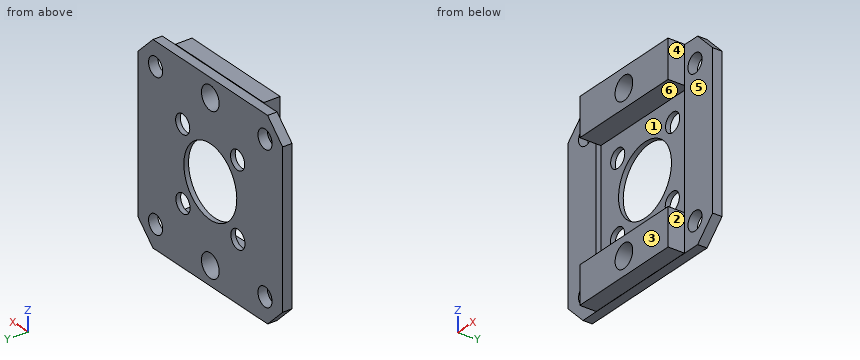
```python
from build123d import *

# Parameters (mm, degrees)
SKETCH2_W           = 41
SKETCH2_H           = 41
BOSS_EXTRUDE1_DEPTH = 2
SKETCH3_R           = 2
CUT_EXTRUDE1_DEPTH  = 30.060282173
SKETCH4_R           = 7.5
CUT_EXTRUDE2_DEPTH  = 30.060282173
SKETCH5_W           = 25
SKETCH5_H           = 25
CUT_EXTRUDE3_DEPTH  = 1
CUT_EXTRUDE4_DEPTH  = 30.060282173
SKETCH7_R           = 2
CUT_EXTRUDE5_DEPTH  = 30.060282173
SKETCH8_W           = 25
SKETCH8_H           = 8.111036271
SKETCH8_H_2         = 7.957817611
BOSS_EXTRUDE2_DEPTH = 3.5
SKETCH9_R           = 2.5
CUT_EXTRUDE6_DEPTH  = 30.585719801


with BuildPart() as part:
    # Sketch2 → Boss-Extrude1 (new body)
    with BuildSketch(Plane(origin=(0, 0, 0), x_dir=(1, 0, 0), z_dir=(0, 1, 0))):
        Rectangle(SKETCH2_W, SKETCH2_H)
    extrude(amount=BOSS_EXTRUDE1_DEPTH)

    # Sketch3 → Cut-Extrude1 (cut, through all)
    with BuildSketch(Plane.XZ):
        with Locations(Location((-7.732300971, 7.823779246, 0), (0, 0, 270))):
            Circle(SKETCH3_R)
        with Locations(Location((7.823779246, 7.732300971, 0), (0, 0, 270))):
            Circle(SKETCH3_R)
        with Locations(Location((7.732300971, -7.823779246, 0), (0, 0, 270))):
            Circle(SKETCH3_R)
        with Locations(Location((-7.823779246, -7.732300971, 0), (0, 0, 270))):
            Circle(SKETCH3_R)
    extrude(amount=-CUT_EXTRUDE1_DEPTH, mode=Mode.SUBTRACT)

    # Sketch4 → Cut-Extrude2 (cut, through all)
    with BuildSketch(Plane(origin=(0, 2, 0), x_dir=(1, 0, 0), z_dir=(0, 1, 0))):
        with Locations(Location((0, 0, 0), (0, 0, 270))):
            Circle(SKETCH4_R)
    extrude(amount=-CUT_EXTRUDE2_DEPTH, mode=Mode.SUBTRACT)

    # Sketch5 → Cut-Extrude3 (cut)
    with BuildSketch(Plane.XZ):
        Rectangle(SKETCH5_W, SKETCH5_H)
    extrude(amount=-CUT_EXTRUDE3_DEPTH, mode=Mode.SUBTRACT)

    # Sketch6 → Cut-Extrude4 (cut, through all)
    with BuildSketch(Plane(origin=(0, 2, 0), x_dir=(1, 0, 0), z_dir=(0, 1, 0))):
        Polygon((-20.5, 16.257359313), (-16.257359313, 20.5), (-20.5, 20.5), align=None)
        Polygon((16.257359313, 20.5), (20.5, 16.257359313), (20.5, 20.5), align=None)
        Polygon((20.5, -16.257359313), (16.257359313, -20.5), (20.5, -20.5), align=None)
        Polygon((-16.257359313, -20.5), (-20.5, -16.257359313), (-20.5, -20.5), align=None)
    extrude(amount=-CUT_EXTRUDE4_DEPTH, mode=Mode.SUBTRACT)

    # Sketch7 → Cut-Extrude5 (cut, through all)
    with BuildSketch(Plane.XZ):
        with Locations(Location((-15.5, 15.5, 0), (0, 0, 270))):
            Circle(SKETCH7_R)
        with Locations(Location((15.5, 15.5, 0), (0, 0, 270))):
            Circle(SKETCH7_R)
        with Locations(Location((15.5, -15.5, 0), (0, 0, 270))):
            Circle(SKETCH7_R)
        with Locations(Location((-15.5, -15.5, 0), (0, 0, 270))):
            Circle(SKETCH7_R)
    extrude(amount=-CUT_EXTRUDE5_DEPTH, mode=Mode.SUBTRACT)

    # Sketch8 → Boss-Extrude2 (add)
    with BuildSketch(Plane.XZ):
        with Locations((0, 16.555518136)):
            Rectangle(SKETCH8_W, SKETCH8_H)
        with Locations((0, -16.478908806)):
            Rectangle(SKETCH8_W, SKETCH8_H_2)
    extrude(amount=BOSS_EXTRUDE2_DEPTH)

    # Sketch9 → Cut-Extrude6 (cut, through all)
    with BuildSketch(Plane.XZ.offset(3.5)):
        with Locations(Location((0, 16.5, 0), (0, 0, 270))):
            Circle(SKETCH9_R)
        with Locations(Location((0, -16.478908806, 0), (0, 0, 270))):
            Circle(SKETCH9_R)
    extrude(amount=-CUT_EXTRUDE6_DEPTH, mode=Mode.SUBTRACT)


solid = part.part
```
The listing builds one solid part. Answer for the finished solid, in the listing's coordinates (mm). Face numbers are marked on the shaded views. A direction names the side the tool comes from. Give positions to 0.01 mm unless a question says otherwise; leave off trailing zeros. Write each loop counter-clockwise with the first axis right and the second up, starting at its lowest first coordinate (ties: lowest second). Pieces come first, ordered by that corner, then holes. Notation, with made-up numbers: (42, 84) -> (51, 84) arc R32 cw to (51, 115) -> close; hole circle Ø1 at (40, 13.25). An arc over 180 degrees is marked (long way). Write item = value, one per line. Start each with the question number.
1) The part is cut by section B-B, the plane x = 0. Determine the outline of the cut face in (y, z), and give its area (3 significant figures).
2) The part is cut by section C-C, the plane x = 15.5. Determine the outline of the cut face in (y, z), and give its area (3 significant figures).
3) Which of the six approach directions +Z, -Z, +X, -X, +Y, -Y give full straight-line access (tool end or side, diameter ignored) to the marked faces 1, 2 and 3?
4) The part is cut by section D-D, the plane z = -12. Determine the outline of the cut face in (x, y), and give its area (3 significant figures).
5) Each of these flat-tipped pins is pushed along its axis until it touches: pin 1 (1.8 mm diameter, centred on x = -5, y = -2, fed in from -Z); pin 2 (6 mm diameter, centred on x = -13, z = -9.5, fed in from -Y); pin 3 (1.8 mm diameter, centred on y = -2, z = 18.5, fed in from -X); pin 4 (3 mm diameter, centred on x = -1.5, z = -15, fed in from +Y). Where does it stop, or does it pass through?
6) Straight lines are drawn through the part: line 1 along Z through (x, y) = (9.5, -1.4); line 2 along X through (y, z) = (-2.15, 16.5); line 3 along X through (y, z) = (0.25, 9). For each, find the intervals that lie inside material, in ascending order.
7) Determine the mould class of the marked faces 4, 5 and 6 for opening direction X: +X half, -X half, draft (parallel to the pull), parting line (faces both ways), or undercut.
8) The part is cut by section A-A, the plane y = -2.1. Determine the outline of the cut face in (x, z).
Solutions:
q1.outline = (-3.5, -20.46) -> (0, -20.46) -> (0, -20.5) -> (2, -20.5) -> (2, -18.98) -> (-3.5, -18.98) -> close; (-3.5, -13.98) -> (2, -13.98) -> (2, -7.5) -> (1, -7.5) -> (1, -12.5) -> (-3.5, -12.5) -> close; (-3.5, 12.5) -> (1, 12.5) -> (1, 7.5) -> (2, 7.5) -> (2, 14) -> (-3.5, 14) -> close; (-3.5, 19) -> (2, 19) -> (2, 20.5) -> (0, 20.5) -> (0, 20.61) -> (-3.5, 20.61) -> close
q1.area = 43.2 mm²
q2.outline = (0, -20.5) -> (2, -20.5) -> (2, -17.5) -> (0, -17.5) -> close; (0, -13.5) -> (2, -13.5) -> (2, 13.5) -> (0, 13.5) -> close; (0, 17.5) -> (2, 17.5) -> (2, 20.5) -> (0, 20.5) -> close
q2.area = 66.0 mm²
q3.face_1 = -Y
q3.face_2 = +Z, -Z, +X, -Y
q3.face_3 = +Z, -Z, +X, -X, -Y
q4.outline = (-20.5, 0) -> (-12.5, 0) -> (-12.5, 1) -> (12.5, 1) -> (12.5, 0) -> (20.5, 0) -> (20.5, 2) -> (-20.5, 2) -> close
q4.area = 57.0 mm²
q5.pin_1 = -20.46
q5.pin_2 = 0
q5.pin_3 = -12.5
q5.pin_4 = 2
q6.line_1 = -20.46 to -12.5, 12.5 to 20.61
q6.line_2 = -12.5 to -2.5, 2.5 to 12.5
q6.line_3 = -20.5 to -12.5, 12.5 to 20.5
q7.face_4 = +X half
q7.face_5 = draft
q7.face_6 = undercut
q8.outline = (-12.5, -20.46) -> (12.5, -20.46) -> (12.5, -12.5) -> (-12.5, -12.5) -> close; (-12.5, 12.5) -> (12.5, 12.5) -> (12.5, 20.61) -> (-12.5, 20.61) -> close; hole circle Ø5 at (0, -16.48); hole circle Ø5 at (0, 16.5)
